CAD build for the part. Positions are in the model's coordinates, mm. A direction names the side the tool comes from. Coordinates: 2 decimals unless noted, no trailing zeros. Loops run counter-clockwise (first coordinate to the right, second up) from the corner with the lowest first, then second, coordinate; pieces in that order, holes last. Notation, with made-up numbers: (17, 40.5) -> (73, 40.5) arc R17 cw to (73, 64.5) -> close; hole circle Ø8 at (-23, 31.5). An arc over 180 degrees is marked (long way). Return JSON: item names as keys, results as strings. Group by question number.
(1) Saw through at D-D on z = 5.75. Write the cut outline in (x, y), then the cut area to 3 significant figures.
(2) Probe L1, parallel to X at y = 45, z = 25.75. List the from-to ranges inside material, lowest first.
(3) Saw through at B-B on z = 15. Write the cut outline in (x, y), then the cut area to 3 significant figures.
(4) Flat gauge pins, fed straight in: pin 1 Ø1 at (y, z) = (63, 17) entering from -X; pin 2 Ø10 at (y, z) = (15.5, 17) entering from +X; pin 3 Ø2 at (x, z) = (29.5, 26) entering from +Y. Where does each tip first touch, or does it go through?
(5) Tool access for faces 5 (the face through (0.57, 0.6, 14.79)), 6 (the face through (45, 1, 11)), 7 (the face through (2, 41, 8)), 8 (the face through (1, 74, 15)), 9 (the face through (0, 42, 8)): list every direction of +Z, -Z, +X, -X, +Y, -Y with a clear straight run to the whole face (end or side of a thin tool).
(6) Saw through at A-A on y = 40. Write the cut outline in (x, z), then the cut area to 3 significant figures.
(7) Mould opens along Y. For faces 1 (the face through (42, 2, 8)), 2 (the face through (1, 50, 19)), 3 (the face through (16, 1, 15)), 4 (the face through (40, 0, 8)) say: pulls with the +Y half, pulls with the -Y half, needs draft (parallel to the pull), parting line crosses it, or undercut.
```python
from build123d import *

# Parameters (mm, degrees)
BOSS_EXTRUDE1_DEPTH = 30
CUT_EXTRUDE1_REACH  = 117.689
CUT_EXTRUDE2_REACH  = 117.689


with BuildPart() as part:
    # Sketch1 → Boss-Extrude1 (new body)
    with BuildSketch(Plane.XY):
        with BuildLine():
            Line((0, 80), (0, 2))
            ThreePointArc((0, 2), (0.585786438, 0.585786438), (2, 0))
            Line((2, 0), (80, 0))
            Line((80, 0), (80, 2))
            Line((80, 2), (2.5, 2))
            ThreePointArc((2.5, 2), (2.146446609, 2.146446609), (2, 2.5))
            Line((2, 2.5), (2, 80))
            Line((2, 80), (0, 80))
        make_face()
    extrude(amount=BOSS_EXTRUDE1_DEPTH)

    # Sketch2 → Cut-Extrude1 (cut, up to next)
    with BuildSketch(Plane(origin=(0, 2, 0), x_dir=(1, 0, 0), z_dir=(0, 1, 0)), mode=Mode.PRIVATE) as cut_extrude1_sk1:
        with BuildLine():
            Line((70, -19), (20, -19))
            ThreePointArc((20, -19), (16, -15), (20, -11))
            Line((20, -11), (70, -11))
            ThreePointArc((70, -11), (74, -15), (70, -19))
        make_face()
    cut_extrude1_tool1 = extrude(cut_extrude1_sk1.sketch, amount=-CUT_EXTRUDE1_REACH, mode=Mode.PRIVATE) & part.part
    add(cut_extrude1_tool1.solids().sort_by_distance((45, 2, 15))[0], mode=Mode.SUBTRACT)

    # Sketch3 → Cut-Extrude2 (cut, up to next)
    with BuildSketch(Plane(origin=(2, 0, 0), x_dir=(0, 0, -1), z_dir=(1, 0, 0)), mode=Mode.PRIVATE) as cut_extrude2_sk1:
        with BuildLine():
            Line((-11, 70), (-11, 30))
            ThreePointArc((-11, 30), (-15, 26), (-19, 30))
            Line((-19, 30), (-19, 70))
            ThreePointArc((-19, 70), (-15, 74), (-11, 70))
        make_face()
    cut_extrude2_tool1 = extrude(cut_extrude2_sk1.sketch, amount=-CUT_EXTRUDE2_REACH, mode=Mode.PRIVATE) & part.part
    add(cut_extrude2_tool1.solids().sort_by_distance((2, 50, 15))[0], mode=Mode.SUBTRACT)


solid = part.part
```
Geometry results:
{
 "1": {"outline": "(0, 2) arc R2 ccw to (2, 0) -> (80, 0) -> (80, 2) -> (2.5, 2) arc R0.5 cw to (2, 2.5) -> (2, 80) -> (0, 80) -> close", "area": "315 mm²"},
 "2": {"L1": "0 to 2"},
 "3": {"outline": "(0, 2) arc R2 ccw to (2, 0) -> (16, 0) -> (16, 2) -> (2.5, 2) arc R0.5 cw to (2, 2.5) -> (2, 26) -> (0, 26) -> close; (0, 74) -> (2, 74) -> (2, 80) -> (0, 80) -> close; (74, 0) -> (80, 0) -> (80, 2) -> (74, 2) -> close", "area": "103 mm²"},
 "4": {"pin 1": "through", "pin 2": "x = 2", "pin 3": "y = 2"},
 "5": {"face 5": "+Z, -Z, -X, -Y", "face 6": "+Y, -Y", "face 7": "+Z, -Z, +X, +Y", "face 8": "+X, -X", "face 9": "+Z, -Z, -X, +Y, -Y"},
 "6": {"outline": "(0, 0) -> (2, 0) -> (2, 11) -> (0, 11) -> close; (0, 19) -> (2, 19) -> (2, 30) -> (0, 30) -> close", "area": "44.0 mm²"},
 "7": {"face 1": "pulls with the +Y half", "face 2": "undercut", "face 3": "needs draft", "face 4": "pulls with the -Y half"}
}
